The model under review builds one solid part; all positions refer to its coordinate system, in mm. Coordinates: 2 decimals unless noted, no trailing zeros. Loops run counter-clockwise (first coordinate to the right, second up) from the corner with the lowest first, then second, coordinate; pieces in that order, holes last. Notation, with made-up numbers: M 71.25,-16.5 L 98.25,-16.5 A16 cw 98.25,-7.5 Z; hole C 17.5,77 d2. An arc over 180 degrees is marked long. Use CSV: the item, a comma, the result in double quotes. Start each with the question number.
1. For L1, parallel to Y at x = 15, z = 1.55; L2, parallel to X at y = 34.5, z = 1.35; L3, parallel to Y at x = 40, z = 2.3, list the stretches that pass through material, from the lowest coordinate up.
2. Add section B-B, the plane y = 20. Write out the cut boundary in (x, z), then the cut area to 3 significant figures.
3. Add section A-A, the plane x = 36.5. Write out the cut boundary in (y, z), then the cut area to 3 significant figures.
4. Clearance check with a flat-ended pin moving along its axis: P1, Ø5, axis at x = 55.5, y = 4.5, coming from the +Z side. State where the tip first meets the part, or that it passes through.
5. Add section C-C, the plane z = 0.6. Write out the cut boundary in (x, y).
6. Draft analysis for pull direction X (two halves, no side actions). For faces 1 (the flat face through (59, 39, 1)), 2 (the flat face through (30, 40, 1)), 3 (the cylindrical face through (13, 5, 2)), state which applies: +X half, -X half, draft (parallel to the pull), parting line (faces both ways), or undercut.
7. Add section D-D, the plane x = 24.5. Write out the cut boundary in (y, z).
from build123d import *

# Parameters (mm, degrees)
SKETCH1_W           = 60
SKETCH1_H           = 40
BOSS_EXTRUDE1_DEPTH = 3
SKETCH2_R           = 2
SKETCH2_R_2         = 12.5
CUT_EXTRUDE1_DEPTH  = 73.173402303
CHAMFER1_SIZE       = 2


with BuildPart() as part:
    # Sketch1 → Boss-Extrude1 (new body)
    with BuildSketch(Plane.XY):
        with Locations((30, 20)):
            Rectangle(SKETCH1_W, SKETCH1_H)
    extrude(amount=BOSS_EXTRUDE1_DEPTH)

    # Sketch2 → Cut-Extrude1 (cut, through all)
    with BuildSketch(Plane.XY.offset(3)):
        with Locations((24.5, 35.5)):
            Circle(SKETCH2_R)
        with Locations((55.5, 35.5)):
            Circle(SKETCH2_R)
        with Locations((55.5, 4.5)):
            Circle(SKETCH2_R)
        with Locations((24.5, 4.5)):
            Circle(SKETCH2_R)
        with Locations((40, 20)):
            Circle(SKETCH2_R_2)
        with Locations((15, 35)):
            Circle(SKETCH2_R)
        with Locations((15, 5)):
            Circle(SKETCH2_R)
    extrude(amount=-CUT_EXTRUDE1_DEPTH, mode=Mode.SUBTRACT)

    # Chamfer1
    chamfer1_edges = [part.edges().sort_by_distance(p)[0] for p in [
        (0, 40, 1.5),
        (60, 40, 1.5),
        (60, 0, 1.5),
        (0, 0, 1.5),
    ]]
    chamfer(chamfer1_edges, length=CHAMFER1_SIZE)


solid = part.part
Computed:
1,L1,"y = 0 to 3, 7 to 33, 37 to 40"
1,L2,"x = 0 to 13.06, 16.94 to 22.77, 26.23 to 53.77, 57.23 to 60"
1,L3,"y = 0 to 7.5, 32.5 to 40"
2,outline,"M 0,0 L 27.5,0 L 27.5,3 L 0,3 Z; M 52.5,0 L 60,0 L 60,3 L 52.5,3 Z"
2,area,"105 mm^2"
3,outline,"M 0,0 L 8,0 L 8,3 L 0,3 Z; M 32,0 L 40,0 L 40,3 L 32,3 Z"
3,area,"48.0 mm^2"
4,P1,"stops at z = 3"
5,outline,"M 0,2 L 2,0 L 58,0 L 60,2 L 60,38 L 58,40 L 2,40 L 0,38 Z; hole C 15,5 d4; hole C 15,35 d4; hole C 24.5,4.5 d4; hole C 24.5,35.5 d4; hole C 40,20 d25; hole C 55.5,4.5 d4; hole C 55.5,35.5 d4"
6,face 1,"+X half"
6,face 2,"draft"
6,face 3,"undercut"
7,outline,"M 0,0 L 2.5,0 L 2.5,3 L 0,3 Z; M 6.5,0 L 33.5,0 L 33.5,3 L 6.5,3 Z; M 37.5,0 L 40,0 L 40,3 L 37.5,3 Z"
